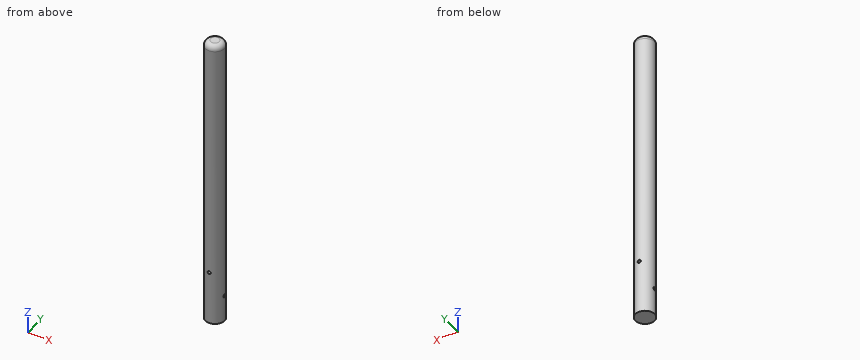
```python
from build123d import *

# Parameters (mm, degrees)
F0_R     = 18
F1_DEPTH = 550
F2_R     = 10
F4_D     = 6
F4_DEPTH = 18.001
F5_D     = 6
F7_D     = 6
F7_DEPTH = 18.0010001
F8_D     = 6


with BuildPart() as f1:
    # F0 (on Top) → F1 (new body)
    with BuildSketch(Plane.XY):
        Circle(F0_R)
    extrude(amount=F1_DEPTH)

    # F2
    f2_edges = [f1.edges().sort_by_distance(p)[0] for p in [
        (-18, 0, 550),
    ]]
    fillet(f2_edges, radius=F2_R)

    # F4 (through all, one way)
    with BuildSketch(Plane(origin=(0, 0, 0), x_dir=(1, 0, 0), z_dir=(0, 1, 0))):
        with Locations((0, -100)):
            Circle(F4_D / 2)
    extrude(amount=-F4_DEPTH, mode=Mode.SUBTRACT)

    # F5 (through all)
    with Locations(Plane.XZ):
        with Locations((0, 100)):
            Hole(F5_D / 2)

    # F7 (through all, one way)
    with BuildSketch(Plane(origin=(0, 0, 0), x_dir=(0, 1, 0), z_dir=(-1, 0, 0))):
        with Locations((0, -50)):
            Circle(F7_D / 2)
    extrude(amount=-F7_DEPTH, mode=Mode.SUBTRACT)

    # F8 (through all)
    with Locations(Plane.YZ):
        with Locations((0, 50)):
            Hole(F8_D / 2)


solid = f1.part
```
Source: CAD feature listing. Evaluate the final solid. Frame: model axes, mm. Round coordinates to 2 decimals unless told otherwise and drop trailing zeros. Loops run counter-clockwise (first coordinate to the right, second up) from the corner with the lowest first, then second, coordinate; pieces in that order, holes last.
1. Ray query, L1, parallel to Z at x = 0, y = 5; L2, parallel to Z at x = 0.5, y = -1; L3, parallel to Y at x = 0.5, z = 232.5. Return the intervals inside material, ascending.
2. Section query A-A on z = 440. Output: boundary loops of the cut face in (x, y), and give its area (3 significant figures).
3. Contact query for flat-ended pins moving along their axis: pin 1 (8 mm diameter, centred on y = -11.5, z = 362.5, fed in from -X); pin 2 (8 mm diameter, centred on x = -11.5, y = 6, fed in from +Z); pin 3 (1 mm diameter, centred on y = -9.5, z = 88, fed in from +X); pin 4 (8 mm diameter, centred on x = 5.5, y = -0.5, fed in from -Z). Output: stop coordinate, or through.
Answers below:
1. L1: z = 0 to 97, 103 to 550
1. L2: z = 0 to 47.17, 52.83 to 97.04, 102.96 to 550
1. L3: y = -17.99 to 17.99
2. outline: circle Ø36 at (0, 0)
2. area: 1,020 mm2
3. pin 1: stops at x = -16.36
3. pin 2: stops at z = 549.95
3. pin 3: stops at x = 15.59
3. pin 4: stops at z = 0
